For this review, take the finished solid that the model builds, in its own axes (mm). A direction names the side the tool comes from. Round coordinates to 2 decimals unless told otherwise and drop trailing zeros. Order: outer loops, then holes, each group sorted by start corner. A loop starts at its lowest first (then second) coordinate and runs counter-clockwise, first axis right, second up. Notation, with made-up numbers: (-14.75, 77) -> (-1.75, 77) arc R20 cw to (-1.75, 112) -> close; hole circle Ø7 at (83, 63.5). An arc over 180 degrees is marked (long way). Use a Markdown table: item, result. Add a question column.
1) Consider section C-C (y = -3). State the section outline as (x, z) points.
2) Draft analysis for pull direction Y (two halves, no side actions). For faces 1 (the face through (32, 0, 6.35)), 2 (the face through (21.58, -9.08, 12.79)), 3 (the face through (7.7, -3.9, 9.7)), state which applies: pulls with the +Y half, pulls with the -Y half, needs draft (parallel to the pull), parting line crosses it, or undercut.
3) Consider section B-B (x = 10). State the section outline as (y, z) points, plus the area to 3 significant figures.
4) Machinability: for faces 4 (the face through (21.58, 9.08, 12.79)), 5 (the face through (24, -12.7, 4)), which of the approach directions +Z, -Z, +X, -X, +Y, -Y give a long, thin tool a straight path to every point of the face, cutting with its end or side? Answer none if there is none.
5) Clearance check with flat-ended pins moving along their axes: P1, Ø1, axis at y = 8, z = 13.5, coming from the -X side; P2, Ø1.5, axis at x = 10.5, z = 11, coming from the -Y side. State where each tip first meets the part, or that it passes through.
6) Wall thickness on line 1 along X through (y, z) = (-2.5, 15.25); line 2 along X through (y, z) = (1.5, 13.5); line 3 along Y through (x, z) = (15.5, 3): over which ranges is each line inside the solid? List them lowest first. Write a range as [from, to].
```python
from build123d import *

# Parameters (mm, degrees)
F1_DEPTH = 12.7
F3_DEPTH = 6.351
F4_R     = 6.35
F5_DEPTH = 19.051
F6_R     = 12.7
F7_R     = 12.69999
F8_R     = 12.69999
F9_R     = 12.7


# Not quite as in the source:
# - a fillet or chamfer is up to 0.001 mm smaller than in the source, because OpenCascade refuses the exact size


with BuildPart() as f1:
    # F0 (on Front) → F1 (new body, symmetric)
    with BuildSketch(Plane.XZ):
        Polygon((0, 19.05), (0, 0), (44.45, 0), (44.45, 6.35), (25.4, 6.35), (25.4, 19.05), align=None)
    extrude(amount=F1_DEPTH, both=True)

    # F2 (on face) → F3 (cut, through all)
    with BuildSketch(Plane.XY.offset(6.35)):
        Polygon((34.925, -12.7), (44.45, -12.7), (44.45, 0), align=None)
    extrude(amount=-F3_DEPTH, mode=Mode.SUBTRACT)

    # F4 (on face) → F5 (cut, through all)
    with BuildSketch(Plane.XY.offset(19.05)):
        with Locations((12.7109484747, 0)):
            Circle(F4_R)
    extrude(amount=-F5_DEPTH, mode=Mode.SUBTRACT)

    # F6
    f6_edges = [f1.edges().sort_by_distance(p)[0] for p in [
        (0, -12.7, 9.525),
    ]]
    fillet(f6_edges, radius=F6_R)

    # F7 (radius 12.7 in the source; OpenCascade refuses exactly that, so slightly less here)
    f7_edges = [f1.edges().sort_by_distance(p)[0] for p in [
        (0, 12.7, 9.525),
    ]]
    fillet(f7_edges, radius=F7_R)

    # F8 (radius 12.7 in the source; OpenCascade refuses exactly that, so slightly less here)
    f8_edges = [f1.edges().sort_by_distance(p)[0] for p in [
        (25.4, -12.7, 12.7),
    ]]
    fillet(f8_edges, radius=F8_R)

    # F9
    f9_edges = [f1.edges().sort_by_distance(p)[0] for p in [
        (25.4, 12.7, 12.7),
    ]]
    fillet(f9_edges, radius=F9_R)


solid = f1.part
```
Results list:
| question | item | result |
|---|---|---|
| 1 | outline | (0.36, 0) -> (7.11, 0) -> (7.11, 19.05) -> (0.36, 19.05) -> close; (18.31, 0) -> (42.2, 0) -> (42.2, 6.35) -> (25.04, 6.35) -> (25.04, 19.05) -> (18.31, 19.05) -> close |
| 2 | face 1 | needs draft |
| 2 | face 2 | pulls with the -Y half |
| 2 | face 3 | undercut |
| 3 | outline | (-12.41, 0) -> (-5.74, 0) -> (-5.74, 19.05) -> (-12.41, 19.05) -> close; (5.74, 0) -> (12.41, 0) -> (12.41, 19.05) -> (5.74, 19.05) -> close |
| 3 | area | 254 mm2 |
| 4 | face 4 | +Z, +X, +Y |
| 4 | face 5 | +Z, -Z, +X, -X, -Y |
| 5 | P1 | x = 2.45 |
| 5 | P2 | y = -12.62 |
| 6 | line 1 | [0.25, 6.87], [18.55, 25.15] |
| 6 | line 2 | [0.09, 6.54], [18.88, 25.31] |
| 6 | line 3 | [-12.7, -5.7], [5.7, 12.7] |
